For this review, use the dimensioned drawing (mm, ordinates from the lowest corner) and the shaded views. A direction names the side the tool comes from. Round coordinates to 2 decimals unless told otherwise and drop trailing zeros. Write each loop counter-clockwise with the first axis right and the second up, starting at its lowest first coordinate (ties: lowest second). Pieces come first, ordered by that corner, then holes. Notation, with made-up numbers: M 25.5,3.5 L 74.5,3.5 A28 ccw 74.5,30.5 Z; hole C 61,42 d11. An arc over 180 degrees is marked long. Use one line per item in the form item = value. Start each with the question number.
Item 1: Add section A-A (y = 31). State the section outline as (x, z) points.
Item 2: For line 1 (Z direction, x = 51, y = 53); line 2 (Z direction, x = 27, y = 36); line 3 (Y direction, x = 30, z = 39), list the stretches that pass through material, from the lowest coordinate up. Write a range as [from, to].
Item 3: Add section C-C (z = 39). State the section outline as (x, y) points.
Item 4: For the marked faces 1 and 2, list the 3-axis set-ups (+Z, -Z, +X, -X, +Y, -Y) from which the entire face can be reached by the end or side of a thin tool; tool diameter is ignored.
Item 5: For P1, Ø10, axis at x = 24.5, y = 50.5, coming from the +Z side; P2, Ø12, axis at y = 49, z = 31.5, coming from the -X side, all flat-tipped, find the tip position at first contact; note any pin that passes through.
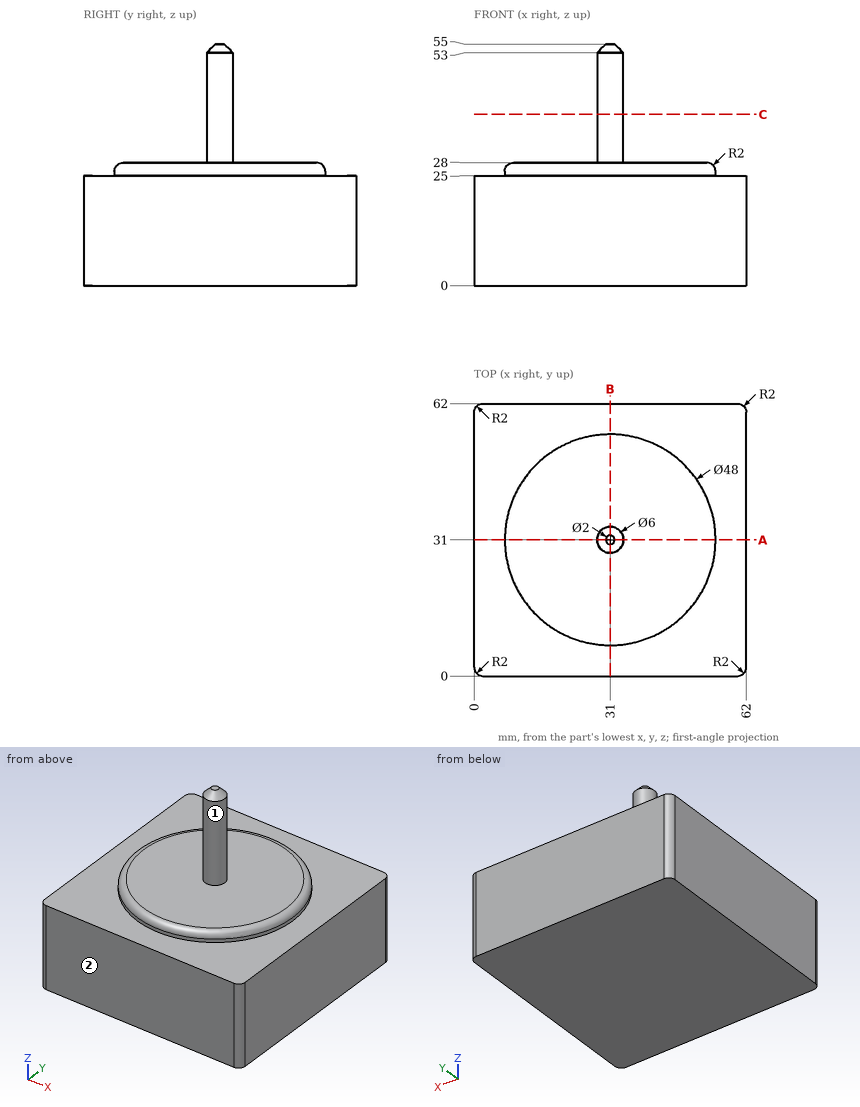
Calculated:
q1.outline = M 0,0 L 62,0 L 62,25 L 55,25 L 55,26 A2 ccw 53,28 L 34,28 L 34,53 L 32,55 L 30,55 L 28,53 L 28,28 L 9,28 A2 ccw 7,26 L 7,25 L 0,25 Z
q2.line_1 = [0, 25]
q2.line_2 = [0, 28]
q2.line_3 = [28.17, 33.83]
q3.outline = C 31,31 d6
q4.face_1 = +Z
q4.face_2 = +Z, -Z, +X, -X, -Y
q5.P1 = 28
q5.P2 = 11.86
